from build123d import *

# Parameters (mm, degrees)
SKETCH_1_R      = 1.5
SKETCH_1_W      = 6
SKETCH_1_H      = 10
EXTRUDE_2_DEPTH = 6


with BuildPart() as part:
    # Эскиз1 → Бобышка-Вытянуть2 (new body)
    with BuildSketch(Plane(origin=(0, 0, 0), x_dir=(1, 0, 0), z_dir=(0, 1, 0))):
        Polygon((-3.416793382, 32.742423734), (5.183206618, 32.742423734), (5.183206618, 22.407164878), (3.146696627, 22.407214255), (3.146623876, 19.406616385), (5.182814398, 19.407762757), (5.184095658, 17.225944952), (7.984095175, 17.227589235), (7.982815638, 19.406473379), (10.020338121, 19.407669902), (10.020410843, 22.407047597), (7.983206618, 22.40709699), (7.983206618, 32.742423734), (16.583206618, 32.742423734), (16.583206618, 38.742423734), (26.583206618, 38.742423734), (26.583206618, 32.742423734), (38.259419898, 32.742423734), (38.255234849, 7.742423734), (-4.416793382, -17.257576266), (-29.416793382, -17.257576266), (-29.416793382, 32.742423734), (-13.416793382, 32.742423734), (-13.416793382, 38.742423734), (-3.416793382, 38.742423734), align=None)
        with Locations((-16.416793382, 7.742423734)):
            Circle(SKETCH_1_R, mode=Mode.SUBTRACT)
        with Locations((-16.416793382, 22.742423734)):
            Rectangle(SKETCH_1_W, SKETCH_1_H, mode=Mode.SUBTRACT)
        with Locations((-16.416793382, -7.257576266)):
            Rectangle(SKETCH_1_W, SKETCH_1_H, mode=Mode.SUBTRACT)
    extrude(amount=EXTRUDE_2_DEPTH)


solid = part.part
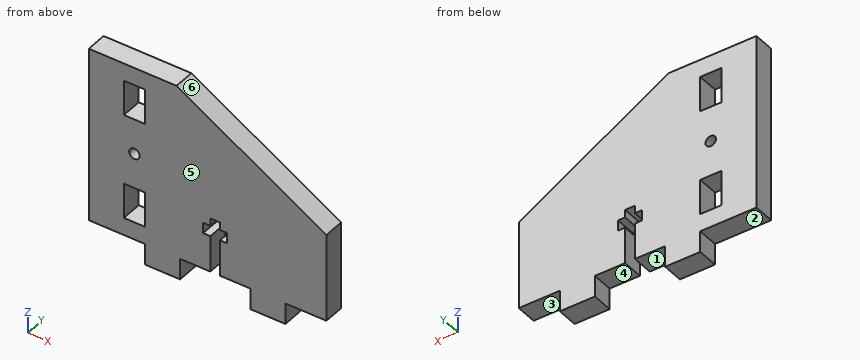
The model under review builds one solid part; all positions refer to its coordinate system, in mm. Face numbers are marked on the shaded views. A direction names the side the tool comes from. Give positions to 0.01 mm unless a question says otherwise; leave off trailing zeros. Loops run counter-clockwise (first coordinate to the right, second up) from the corner with the lowest first, then second, coordinate; pieces in that order, holes last. Notation, with made-up numbers: (49, 25.5) -> (90, 25.5) arc R34 cw to (90, 60.5) -> close; hole circle Ø8 at (49, -32). An arc over 180 degrees is marked (long way). Put each result on its own line as item: value. Start each with the question number.
1. We need section D-D on z = 4. State the section outline as (x, y) points, then the cut area to 3 significant figures.
2. We need section B-B on x = 9. State the section outline as (y, z) points, then the cut area to 3 significant figures.
3. We need section C-C on z = -26.5. State the section outline as (x, y) points.
4. For the marked faces 1, 2 and 3, list the 3-axis set-ups (+Z, -Z, +X, -X, +Y, -Y) from which the entire face can be reached by the end or side of a thin tool; tool diameter is ignored.
5. Mouldability with a two-part tool opening along X and no side actions: class the marked faces 4, 5 and 6 as released by +X, released by -X, zero draft, split by the parting line, or undercut.
6. We need section A-A on y = 3. State how many separate pieces and enclosed holes the cut face has, then the cut area to 3 significant figures.
7. Wall thickness on probe 1 along Z at (x, y) = (-16.5, 5.3); probe 2 along X at (y, z) = (3.05, -20.5); probe 3 along X at (y, z) = (4.2, -18): over which ranges is each line inside the solid? List them lowest first.
8. Clearance check with flat-ended pins moving along their axes: P1, Ø1, axis at y = 4, z = -7, coming from the +X side; P2, Ø3, axis at x = 0.5, y = 4.5, coming from the -Z side; P3, Ø1.6, axis at x = 4, y = 2, coming from the +Z side; P4, Ø2, axis at x = -6, z = -10, coming from the -Y side. State where each tip first meets the part, or that it passes through.
Determined:
1. outline: (-29.42, 0) -> (-19.42, 0) -> (-19.42, 6) -> (-29.42, 6) -> close; (-13.42, 0) -> (18.21, 0) -> (18.21, 6) -> (-13.42, 6) -> close
1. area: 250 mm^2
2. outline: (0, -32.74) -> (6, -32.74) -> (6, -22.41) -> (0, -22.41) -> close; (0, -19.41) -> (6, -19.41) -> (6, 9.4) -> (0, 9.4) -> close
2. area: 235 mm^2
3. outline: (-29.42, 0) -> (-19.42, 0) -> (-19.42, 6) -> (-29.42, 6) -> close; (-13.42, 0) -> (5.18, 0) -> (5.18, 6) -> (-13.42, 6) -> close; (7.98, 0) -> (38.26, 0) -> (38.26, 6) -> (7.98, 6) -> close
4. face 1: -Z, +Y, -Y
4. face 2: -Z, -X, +Y, -Y
4. face 3: -Z, +X, +Y, -Y
5. face 4: undercut
5. face 5: zero draft
5. face 6: released by +X
6. separate pieces: 1
6. enclosed holes: 3
6. area: 2,790 mm^2
7. probe 1: -32.74 to -27.74, -17.74 to -9.24, -6.24 to 2.26, 12.26 to 17.26
7. probe 2: -29.42 to -19.42, -13.42 to 3.15, 10.02 to 38.26
7. probe 3: -29.42 to -19.42, -13.42 to 5.18, 7.98 to 38.26
8. P1: x = 37.84
8. P2: z = -32.74
8. P3: z = 12.8
8. P4: y = 0
